Here's how the part is built. I have some questions about the finished solid (model axes, mm). A direction names the side the tool comes from. Round coordinates to 2 decimals unless told otherwise and drop trailing zeros. Order: outer loops, then holes, each group sorted by start corner. A loop starts at its lowest first (then second) coordinate and runs counter-clockwise, first axis right, second up. Notation, with made-up numbers: (15, -2.75) - (63, -2.75) arc R29 cw to (63, 25.25) - close; hole circle Ø8 at (51, -37.5). An arc over 180 degrees is marked (long way). One line per item, written item: value.
from build123d import *

# Parameters (mm, degrees)
ESQUISSE3_R         = 27.5
ESQUISSE3_R_2       = 1.625
ESQUISSE3_R_3       = 7.6
BOSS_EXTRU_1_DEPTH  = 6.35
ESQUISSE4_R         = 10.5
ESQUISSE4_R_2       = 7.6
BOSS_EXTRU_2_DEPTH  = 45
SKETCH1_R           = 10.5
SKETCH1_R_2         = 4.375
BOSS_EXTRUDE1_DEPTH = 7
SKETCH2_R           = 2.05
CUT_EXTRUDE1_DEPTH  = 6
CHAMFER2_SIZE       = 5.712592027
CHAMFER2_SIZE_2     = 4
CHAMFER3_SIZE       = 2
CHAMFER3_SIZE2      = 1.349017034
SKETCH3_R           = 2.075
CUT_EXTRUDE2_DEPTH  = 8


with BuildPart() as part:
    # Esquisse3 → Boss.-Extru.1 (new body)
    with BuildSketch(Plane.XY):
        Circle(ESQUISSE3_R)
        with Locations((-19.485571585, 11.25)):
            Circle(ESQUISSE3_R_2, mode=Mode.SUBTRACT)
        with Locations((19.485571585, 11.25)):
            Circle(ESQUISSE3_R_2, mode=Mode.SUBTRACT)
        with Locations((0, -22.5)):
            Circle(ESQUISSE3_R_2, mode=Mode.SUBTRACT)
        Circle(ESQUISSE3_R_3, mode=Mode.SUBTRACT)
    extrude(amount=BOSS_EXTRU_1_DEPTH)

    # Esquisse4 → Boss.-Extru.2 (add)
    with BuildSketch(Plane.XY.offset(6.35)):
        with Locations(Location((0, 0, 0), (0, 0, 180))):
            Circle(ESQUISSE4_R)
        Circle(ESQUISSE4_R_2, mode=Mode.SUBTRACT)
    extrude(amount=BOSS_EXTRU_2_DEPTH)

    # Sketch1 → Boss-Extrude1 (add)
    with BuildSketch(Plane.XY.offset(51.35)):
        with Locations(Location((0, 0, 0), (0, 0, 180))):
            Circle(SKETCH1_R)
        Circle(SKETCH1_R_2, mode=Mode.SUBTRACT)
    extrude(amount=BOSS_EXTRUDE1_DEPTH)

    # Sketch2 → Cut-Extrude1 (cut)
    with BuildSketch(Plane.XY.offset(58.35)):
        with Locations((0, 7.5)):
            Circle(SKETCH2_R)
        with Locations((-6.495190528, -3.75)):
            Circle(SKETCH2_R)
        with Locations((6.495190528, -3.75)):
            Circle(SKETCH2_R)
    extrude(amount=-CUT_EXTRUDE1_DEPTH, mode=Mode.SUBTRACT)

    # Chamfer2
    # the kernel refuses this chamfer: 5.712592027, 4 mm, written as the material it adds along each edge
    with BuildSketch(Plane(origin=(0, 0, 51.35), x_dir=(1, 0, 0), z_dir=(0, -1, 0))) as chamfer2_piece_1_section:
        Polygon((7.6, -CHAMFER2_SIZE), (7.6 - CHAMFER2_SIZE_2, 0), (7.6, 0), align=None)
    chamfer2_piece_1 = revolve(axis=Axis((0, 0, 51.35), (0, 0, 1)), mode=Mode.PRIVATE)
    chamfer2_piece_1 = chamfer2_piece_1 - Plane(origin=(0, 0, 47.891956694), x_dir=(1, 0, 0), z_dir=(0, 0, -1)) * Cylinder(4.375, 31, mode=Mode.PRIVATE)
    add(chamfer2_piece_1)

    # Chamfer3
    chamfer3_edges = [part.edges().sort_by_distance(p)[0] for p in [
        (10.5, 0, 6.35),
    ]]
    chamfer3_side = [part.faces().sort_by_distance(p)[0] for p in [
        (-26.722182541, 0, 6.35),
    ]]
    chamfer(chamfer3_edges, length=CHAMFER3_SIZE, length2=CHAMFER3_SIZE2, reference=chamfer3_side[0])

    # Sketch3 → Cut-Extrude2 (cut)
    with BuildSketch(Plane.XY.offset(6.35)):
        with Locations((0, 17.5)):
            Circle(SKETCH3_R)
        with Locations((-15.155444566, -8.75)):
            Circle(SKETCH3_R)
        with Locations((15.155444566, -8.75)):
            Circle(SKETCH3_R)
    extrude(amount=-CUT_EXTRUDE2_DEPTH, mode=Mode.SUBTRACT)


solid = part.part
Q1. If we section it at A-A, the plane x = 0: Give the number of separate pieces and of enclosed holes in the cut face, then the cut area to 3 significant figures.
Results list:
separate pieces: 4
enclosed holes: 0
area: 553 mm²
Q2. If we section it at B-B, the plane y = 0: Please give me the cut outline in (x, z) (3 decimals).
Results list:
outline: (-27.5, 0) - (-7.6, 0) - (-7.6, 45.637) - (-4.375, 50.243) - (-4.375, 58.35) - (-10.5, 58.35) - (-10.5, 7.699) - (-12.5, 6.35) - (-27.5, 6.35) - close; (4.375, 50.243) - (7.6, 45.637) - (7.6, 0) - (27.5, 0) - (27.5, 6.35) - (12.5, 6.35) - (10.5, 7.699) - (10.5, 58.35) - (4.375, 58.35) - close
Q3. If we section it at C-C, the plane x = -14: Please give me the cut outline in (y, z), then the cut area to 3 significant figures.
Results list:
outline: (-23.67, 0) - (-10.47, 0) - (-10.47, 6.35) - (-23.67, 6.35) - close; (-7.03, 0) - (23.67, 0) - (23.67, 6.35) - (-7.03, 6.35) - close
area: 279 mm²
Q4. If I drill on line 1 along Y through (x, z) = (0, 56) (3 decimals); line 2 along Z through (x, y) = (-18, -11.5); line 3 along X through (y, z) = (11.5, 3), over which ranges is the centre line in solid material (lowest first)?
Results list:
line 1: -10.5 to -4.375, 4.375 to 5.45, 9.55 to 10.5
line 2: 0 to 6.35
line 3: -24.98 to -21.09, -17.88 to 17.88, 21.09 to 24.98
Q5. Will these pins go through, and if not, where does the flat tip stop? pin 1 (1 mm diameter, centred on x = -1.5, y = -4.5, fed in from -Z); pin 2 (7 mm diameter, centred on x = 0, y = 0, fed in from +Z); pin 3 (2.5 mm diameter, centred on x = -6.5, y = -3.75, fed in from +Z); pin 4 (10 mm diameter, centred on x = -12, z = 29.5, fed in from +Y).
Results list:
pin 1: z = 49
pin 2: through
pin 3: z = 52.35
pin 4: y = 7.83
Q6. We'd pull the mould along Y, two halves only. Please class faces 3 (the cylindrical face through (-0.444, 5.499, 55.392)), 4 (the cylindrical face through (-10, -3.2, 32.7)), 5 (the flat face through (12, -6, 6.35)): released by +Y, released by -Y, zero draft, split by the parting line, or undercut.
Results list:
face 3: undercut
face 4: split by the parting line
face 5: zero draft
Q7. Which directions (+Z, -Z, +X, -X, +Y, -Y) give clear straight access to the entire face, cutting with the end or side of a thin tool? Please do faces 1 (the flat face through (-7, -4, 52.35)), 2 (the flat face through (6, -6, 0)).
Results list:
face 1: +Z
face 2: -Z, +X, -X, +Y, -Y
Q8. If we section it at D-D, the plane z = 41: Please give me the cut outline in (x, y), then the cut area to 3 significant figures.
Results list:
outline: circle Ø21 at (0, 0); hole circle Ø15.2 at (0, 0)
area: 165 mm²
